from build123d import *

# Parameters (mm, degrees)
BOSS_EXTRUDE1_DEPTH = 22
SKETCH2_R           = 5
BOSS_EXTRUDE2_DEPTH = 11
SKETCH3_R           = 3
CUT_EXTRUDE1_DEPTH  = 11


with BuildPart() as part:
    # Sketch1 → Boss-Extrude1 (new body)
    with BuildSketch(Plane(origin=(0, 0, 0), x_dir=(0, 0, -1), z_dir=(1, 0, 0))):
        Polygon((2.396003617, -4.15), (4.792007234, 0), (2.396003617, 4.15), (-2.396003617, 4.15), (-4.792007234, 0), (-2.396003617, -4.15), align=None)
    extrude(amount=BOSS_EXTRUDE1_DEPTH)

    # Sketch2 → Boss-Extrude2 (add)
    with BuildSketch(Plane.ZY):
        Circle(SKETCH2_R)
    extrude(amount=BOSS_EXTRUDE2_DEPTH)

    # Sketch3 → Cut-Extrude1 (cut)
    with BuildSketch(Plane.ZY.offset(11)):
        Circle(SKETCH3_R)
    extrude(amount=-CUT_EXTRUDE1_DEPTH, mode=Mode.SUBTRACT)


solid = part.part
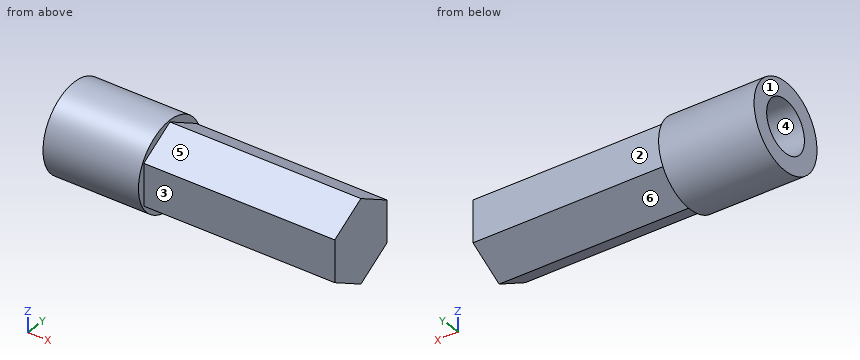
The model under review builds one solid part; all positions refer to its coordinate system, in mm. Face numbers are marked on the shaded views. A direction names the side the tool comes from. Round coordinates to 2 decimals unless told otherwise and drop trailing zeros. Write each loop counter-clockwise with the first axis right and the second up, starting at its lowest first coordinate (ties: lowest second). Pieces come first, ordered by that corner, then holes. Notation, with made-up numbers: M -27,80 L 30,80 A29 cw 30,101 Z; hole C 13.25,29.5 d3. An arc over 180 degrees is marked long. Use a Markdown table: item, result. Add a question column.
Q1. Insertion check: pin 1 (5.5 mm diameter, centred on x = 11.5, z = 0, fed in from +Y); pin 2 (3 mm diameter, centred on x = 4, z = -2.5, fed in from -Y); pin 3 (1 mm diameter, centred on x = -2, y = 3, fed in from +Z). Each pin has a flat end and moves straight along its axis. Give the tip position at first contact, or say it passes through.
Q2. The part is to be moulded in two halves that separate along Z. For the marked faces 4, 5 and 6, say which applies: pulls with the +Z half, pulls with the -Z half, needs draft (parallel to the pull), parting line crosses it, or undercut.
Q3. We need section D-D, the plane z = -4. State the section outline as (x, y) points.
Q4. We need section B-B, the plane x = 10. State the section outline as (y, z) points.
Q5. We need section A-A, the plane z = 0. State the section outline as (x, y) points, plus the area to 3 significant figures.
Q6. We need section C-C, the plane y = 2. State the section outline as (x, z) points.
Q7. Machinability: for the marked faces 1, 2 and 3, which of the approach directions +Z, -Z, +X, -X, +Y, -Y give a long, thin tool a straight path to every point of the face, cutting with its end or side? Answer none if there is none.
Q8. To check wall thickness, follow line 1 (Y direction, x = -8, z = 0); line 2 (X direction, y = -0.5, z = 2); line 3 (Y direction, x = 1, z = -2). State the ranges of each line that lie inside material, in increasing order.
Findings below:
| question | item | result |
|---|---|---|
| 1 | pin 1 | stops at y = 4.15 |
| 1 | pin 2 | stops at y = -4.15 |
| 1 | pin 3 | stops at z = 4.33 |
| 2 | face 4 | undercut |
| 2 | face 5 | pulls with the +Z half |
| 2 | face 6 | pulls with the -Z half |
| 3 | outline | M -11,-3 L 0,-3 L 0,-1.37 L 22,-1.37 L 22,1.37 L 0,1.37 L 0,3 L -11,3 Z |
| 4 | outline | M -4.15,-2.4 L 0,-4.79 L 4.15,-2.4 L 4.15,2.4 L 0,4.79 L -4.15,2.4 Z |
| 5 | outline | M -11,-5 L 0,-5 L 0,-4.15 L 22,-4.15 L 22,4.15 L 0,4.15 L 0,5 L -11,5 L -11,3 L 0,3 L 0,-3 L -11,-3 Z |
| 5 | area | 227 mm² |
| 6 | outline | M -11,-4.58 L 0,-4.58 L 0,-3.64 L 22,-3.64 L 22,3.64 L 0,3.64 L 0,4.58 L -11,4.58 L -11,2.24 L 0,2.24 L 0,-2.24 L -11,-2.24 Z |
| 7 | face 1 | +Z, -Z, -X, +Y, -Y |
| 7 | face 2 | +Z, -Z, +X, +Y |
| 7 | face 3 | +Z, -Z, +X, -Y |
| 8 | line 1 | y = -5 to -3, 3 to 5 |
| 8 | line 2 | x = 0 to 22 |
| 8 | line 3 | y = -4.15 to 4.15 |
